from build123d import *

# Parameters (mm, degrees)
SKETCH1_W           = 203.2
SKETCH1_H           = 83.82
BOSS_EXTRUDE1_DEPTH = 55.118
CUT_EXTRUDE1_DEPTH  = 227.614267697


with BuildPart() as part:
    # Sketch1 → Boss-Extrude1 (new body)
    with BuildSketch(Plane.XY):
        with Locations((101.6, -41.91)):
            Rectangle(SKETCH1_W, SKETCH1_H)
    extrude(amount=BOSS_EXTRUDE1_DEPTH)

    # Sketch2 → Cut-Extrude1 (cut, through all)
    with BuildSketch(Plane(origin=(203.2, 0, 0), x_dir=(0, 0, -1), z_dir=(1, 0, 0))):
        Polygon((-19.558, -83.82), (-19.558, -81.28), (-52.578, -81.28), (-52.578, -2.54), (0, -2.54), (0, -83.82), align=None)
    extrude(amount=-CUT_EXTRUDE1_DEPTH, mode=Mode.SUBTRACT)


solid = part.part
CAD build for the part. Positions are in the model's coordinates, mm. A direction names the side the tool comes from. Give positions to 0.01 mm unless a question says otherwise; leave off trailing zeros. Order: outer loops, then holes, each group sorted by start corner. A loop starts at its lowest first (then second) coordinate and runs counter-clockwise, first axis right, second up. Notation, with made-up numbers: (-0.75, 73) - (8.25, 73) arc R24 ccw to (8.25, 93) - close; hole circle Ø7 at (71, 71.5). An arc over 180 degrees is marked (long way). Answer in a Markdown table with one row per item.
1. Tool access for faces 1 (the flat face through (100, -83.82, 37)), 2 (the flat face through (103, -42, 52.578)): list every direction of +Z, -Z, +X, -X, +Y, -Y with a clear straight run to the whole face (end or side of a thin tool).
Data:
| item | result |
|---|---|
| face 1 | +Z, -Z, +X, -X, -Y |
| face 2 | -Z, +X, -X |
2. Pull direction Y, two halves, no side cores. Call faces 3 (the flat face through (100, 0, 27)), 4 (the flat face through (100, -41, 55.118)), 5 (the flat face through (103, -2.54, 27)): pulls with the +Y half, pulls with the -Y half, needs draft (parallel to the pull), parting line crosses it, or undercut.
Data:
| item | result |
|---|---|
| face 3 | pulls with the +Y half |
| face 4 | needs draft |
| face 5 | undercut |
3. Saw through at B-B, the plane x = 152. Give the cut face in (y, z), plus the area to 3 significant figures.
Data:
| item | result |
|---|---|
| outline | (-83.82, 19.56) - (-81.28, 19.56) - (-81.28, 52.58) - (-2.54, 52.58) - (-2.54, 0) - (0, 0) - (0, 55.12) - (-83.82, 55.12) - close |
| area | 430 mm² |
4. Saw through at A-A, the plane z = 48. Give the cut face in (x, y), plus the area to 3 significant figures.
Data:
| item | result |
|---|---|
| outline | (0, -83.82) - (203.2, -83.82) - (203.2, -81.28) - (0, -81.28) - close; (0, -2.54) - (203.2, -2.54) - (203.2, 0) - (0, 0) - close |
| area | 1,030 mm² |
5. Probe probe 1 along Y at (x, z) = (56, 47); probe 2 along Z at (x, y) = (43, -12); probe 3 along Y at (x, z) = (10.5, 5.5). List the from-to ranges inside material, lowest first. Write a range as [from, to].
Data:
| item | result |
|---|---|
| probe 1 | y = [-83.82, -81.28], [-2.54, 0] |
| probe 2 | z = [52.58, 55.12] |
| probe 3 | y = [-2.54, 0] |
6. Saw through at D-D, the plane z = 13.5. Give the cut face in (x, y), plus the area to 3 significant figures.
Data:
| item | result |
|---|---|
| outline | (0, -2.54) - (203.2, -2.54) - (203.2, 0) - (0, 0) - close |
| area | 516 mm² |
7. Flat gauge pins, fed straight in: pin 1 (5 mm diameter, centred on x = 167, z = 47, fed in from +Y); pin 2 (10 mm diameter, centred on x = 149.5, y = -70.5, fed in from -Z); pin 3 (3 mm diameter, centred on x = 105, y = -83, fed in from -Z); pin 4 (2 mm diameter, centred on x = 32.5, z = 12.5, fed in from -Y). Where does each tip first touch, or does it go through?
Data:
| item | result |
|---|---|
| pin 1 | stops at y = 0 |
| pin 2 | stops at z = 52.58 |
| pin 3 | stops at z = 19.56 |
| pin 4 | stops at y = -2.54 |
8. Saw through at C-C, the plane y = -47. Give the cut face in (x, z).
Data:
| item | result |
|---|---|
| outline | (0, 52.58) - (203.2, 52.58) - (203.2, 55.12) - (0, 55.12) - close |
